Check sheet for the modelled part. Datum: model origin and axes. Units: mm. Give positions to 0.01 mm unless a question says otherwise; leave off trailing zeros. Loops run counter-clockwise (first coordinate to the right, second up) from the corner with the lowest first, then second, coordinate; pieces in that order, holes last. Notation, with made-up numbers: M 80,-25.5 L 113,-25.5 A21 cw 113,-3.5 Z; hole C 66,56 d10. An arc over 180 degrees is marked long. Write each question's results on one line, items separated by ' | '. Start each with the question number.
1. Go/stop test with flat-tipped pins: pin 1 (2 mm diameter, centred on x = 10, y = 35.5, fed in from +Z) (3 decimals); pin 2 (1 mm diameter, centred on x = 9, z = 3, fed in from +Y); pin 3 (2 mm diameter, centred on y = 76, z = 1, fed in from -X). Record where each tip stops, or that it passes through.
2. Sectioned sample at B-B on x = 4. Record the cut outline in (y, z) (3 decimals).
3. Sectioned sample at C-C on y = 89. Record the cut outline in (x, z) (3 decimals).
4. Sectioned sample at A-A on z = 2.75. Record the cut outline in (x, y).
5. Material ranges on line 1 along Z through (x, y) = (10, 86.5) (3 decimals); line 2 along Y through (x, z) = (3.5, 2.2); line 3 along Y through (x, z) = (3, 4.55), recorded low to high.
```python
from build123d import *

# Parameters (mm, degrees)
F0_W     = 15.24
F0_H     = 7.62
F1_DEPTH = 5.08
F2_W     = 12.7
F2_H     = 1.905
F3_DEPTH = 5.08
F5_DEPTH = 1.905


# Not quite as in the source:
# - a feature names something its author has since deleted; it is built from what else it names


with BuildPart() as f1:
    # F0 (on Top) → F1 (new body)
    with BuildSketch(Plane.XY):
        with Locations((7.62, 3.81)):
            Rectangle(F0_W, F0_H)
    extrude(amount=F1_DEPTH)

    # F2 (on face) → F3 (cut, through all)
    with BuildSketch(Plane(origin=(0, 7.62, 0), x_dir=(-1, 0, 0), z_dir=(0, 1, 0))):
        with Locations((-7.62, 2.8575)):
            Rectangle(F2_W, F2_H)
    extrude(amount=-F3_DEPTH, mode=Mode.SUBTRACT)

    # F4 (on face) → F5 (join, through all)
    with BuildSketch(Plane(origin=(0, 0, 0), x_dir=(1, 0, 0), z_dir=(0, 0, -1))):
        with BuildLine():
            ThreePointArc((10.16, -18.9792253257), (10.7132695997, -16.3868486813), (12.2766666667, -14.2462147733))
            ThreePointArc((12.2766666667, -14.2462147733), (14.4654225604, -11.2493273022), (15.24, -7.62))
            Line((15.24, -7.62), (7.62, -7.62))
            Line((7.62, -7.62), (7.62, -121.92))
            Line((7.62, -121.92), (10.16, -121.92))
            Line((10.16, -121.92), (10.16, -18.9792253257))
        make_face()
    extrude(amount=-F5_DEPTH)

    # F6: F1 across face


with BuildPart() as f1_1:
    add(f1.part)
    add(f1.part.mirror(Plane(origin=(7.62, 64.77, 0.9525), x_dir=(0, -1, 0), z_dir=(-1, 0, 0))))


solid = f1_1.part
```
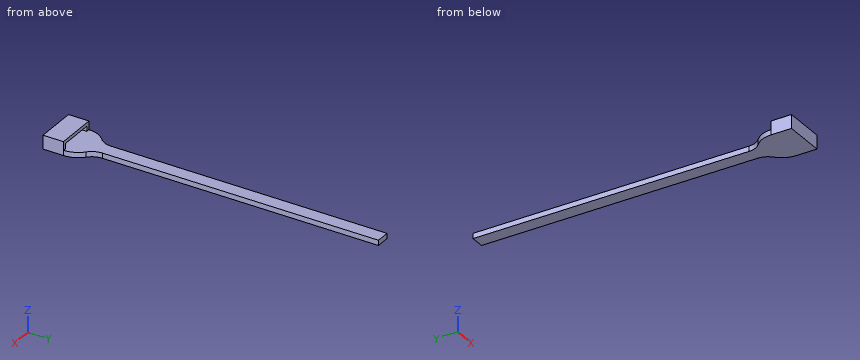
Output values:
1) pin 1: z = 1.905 | pin 2: y = 2.54 | pin 3: x = 5.08
2) outline: M 0,0 L 15.437,0 L 15.437,1.905 L 2.54,1.905 L 2.54,3.81 L 7.62,3.81 L 7.62,5.08 L 0,5.08 Z
3) outline: M 5.08,0 L 10.16,0 L 10.16,1.905 L 5.08,1.905 Z
4) outline: M 0,0 L 15.24,0 L 15.24,7.62 L 13.97,7.62 L 13.97,2.54 L 1.27,2.54 L 1.27,7.62 L 0,7.62 Z
5) line 1: 0 to 1.905 | line 2: 0 to 2.54 | line 3: 0 to 7.62
